Source: CAD feature listing. Evaluate the final solid. Frame: model axes, mm. Face numbers are marked on the shaded views. A direction names the side the tool comes from. Coordinates: 2 decimals unless noted, no trailing zeros. Loops run counter-clockwise (first coordinate to the right, second up) from the corner with the lowest first, then second, coordinate; pieces in that order, holes last. Notation, with made-up numbers: (20.5, -9.75) -> (60.5, -9.75) arc R13 ccw to (60.5, 9.25) -> close; hole circle Ø2 at (-5.75, 23). An arc over 180 degrees is marked (long way). Answer as a JSON object with one key per item and string values. Group by question number.
from build123d import *

# Parameters (mm, degrees)
F0_W     = 35
F0_H     = 35
F1_DEPTH = 10
F2_W     = 18.406059
F2_H     = 20.067719
F3_DEPTH = 25
F4_R     = 5


with BuildPart() as f1:
    # F0 (on Top) → F1 (new body)
    with BuildSketch(Plane.XY):
        with Locations((-30.465538, 24.800614)):
            Rectangle(F0_W, F0_H)
    extrude(amount=F1_DEPTH)

    # F2 (on Top) → F3 (cut)
    with BuildSketch(Plane.XY):
        with Locations((-30.214937, 24.916981)):
            Rectangle(F2_W, F2_H)
    extrude(amount=F3_DEPTH, mode=Mode.SUBTRACT)

    # F4
    f4_edges = [f1.edges().sort_by_distance(p)[0] for p in [
        (-12.965538, 42.300614, 5),
        (-47.965538, 42.300614, 5),
        (-47.965538, 7.300614, 5),
        (-12.965538, 7.300614, 5),
        (-21.011908, 14.883122, 5),
        (-39.417967, 14.883122, 5),
        (-39.417967, 34.950841, 5),
        (-21.011908, 34.950841, 5),
    ]]
    fillet(f4_edges, radius=F4_R)


solid = f1.part
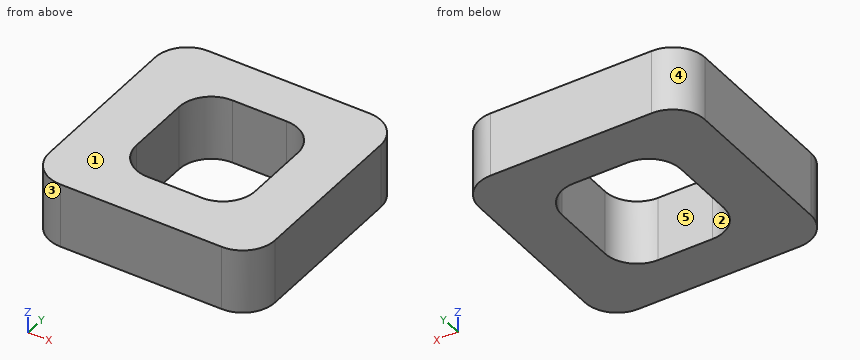
1. Ray query, L1, parallel to X at y = 23, z = 6.25; L2, parallel to Y at x = -28, z = 8.5; L3, parallel to Y at x = -36, z = 3. Return the intervals inside material, ascending.
2. Section query A-A on x = -29.5. Return loops of the section in (y, z).
3. Reachability of the marked faces 4 and 5 from +Z, -Z, +X, -X, +Y, -Y: full face, straight path, thin tool, end or side. Return the list, or none.
4. Mould query, pull axis X, two halves, no side actions, for the marked faces 1, 2 and 3. Classes: pulls with the +X half, pulls with the -X half, needs draft (parallel to the pull), parting line crosses it, or undercut.
5. Section query B-B on y = 29.5. Return loops of the section in (x, z), then the cut area to 3 significant figures.
6. Section query C-C on z = 4.75. Return loops of the section in (x, y), then the cut area to 3 significant figures.
Solved:
{
 "1": {"L1": "-47.97 to -39.42, -21.01 to -12.97", "L2": "7.3 to 14.88, 34.95 to 42.3", "L3": "7.3 to 15.14, 34.69 to 42.3"},
 "2": {"outline": "(7.3, 0) -> (14.88, 0) -> (14.88, 10) -> (7.3, 10) -> close; (34.95, 0) -> (42.3, 0) -> (42.3, 10) -> (34.95, 10) -> close"},
 "3": {"face 4": "+Z, -Z, -X, +Y", "face 5": "+Z, -Z"},
 "4": {"face 1": "needs draft", "face 2": "undercut", "face 3": "pulls with the -X half"},
 "5": {"outline": "(-47.97, 0) -> (-39.42, 0) -> (-39.42, 10) -> (-47.97, 10) -> close; (-21.01, 0) -> (-12.97, 0) -> (-12.97, 10) -> (-21.01, 10) -> close", "area": "166 mm^2"},
 "6": {"outline": "(-47.97, 12.3) arc R5 ccw to (-42.97, 7.3) -> (-17.97, 7.3) arc R5 ccw to (-12.97, 12.3) -> (-12.97, 37.3) arc R5 ccw to (-17.97, 42.3) -> (-42.97, 42.3) arc R5 ccw to (-47.97, 37.3) -> close; hole (-39.42, 19.88) arc R5 ccw to (-34.42, 14.88) -> (-26.01, 14.88) arc R5 ccw to (-21.01, 19.88) -> (-21.01, 29.95) arc R5 ccw to (-26.01, 34.95) -> (-34.42, 34.95) arc R5 ccw to (-39.42, 29.95) -> close", "area": "856 mm^2"}
}
